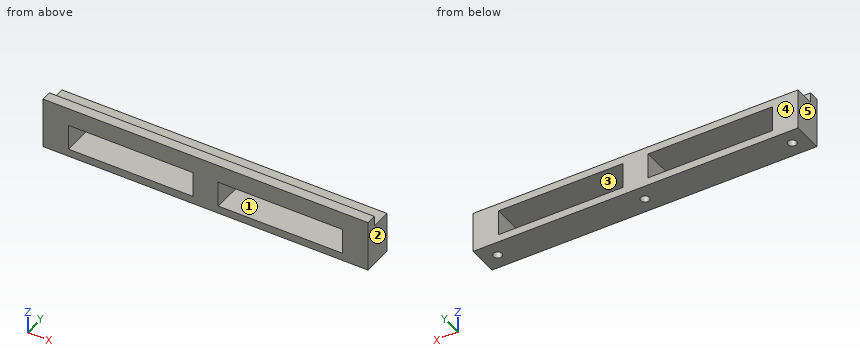
```python
from build123d import *

# Parameters (mm, degrees)
F0_W     = 101.6
F0_H     = 9.525
F1_DEPTH = 12.762509
F2_W     = 101.6
F2_H     = 3.175
F3_DEPTH = 3.175
F4_W     = 38.89375
F4_H     = 8.000009
F5_DEPTH = 9.525
F6_R     = 1.35255
F7_DEPTH = 10.381259


with BuildPart() as f1:
    # F0 (on Top) → F1 (new body)
    with BuildSketch(Plane.XY):
        with Locations((50.8, -4.7625)):
            Rectangle(F0_W, F0_H)
    extrude(amount=F1_DEPTH)

    # F2 (on face) → F3 (join)
    with BuildSketch(Plane.XY.offset(12.762509)):
        with Locations((50.8, -7.9375)):
            Rectangle(F2_W, F2_H)
    extrude(amount=F3_DEPTH)

    # F4 (on face) → F5 (cut, through all)
    with BuildSketch(Plane(origin=(0, 0, 0), x_dir=(-1, 0, 0), z_dir=(0, 1, 0))):
        with Locations((-74.215625, 6.381254)):
            Rectangle(F4_W, F4_H)
        with Locations((-27.384375, 6.381254)):
            Rectangle(F4_W, F4_H)
    extrude(amount=-F5_DEPTH, mode=Mode.SUBTRACT)

    # F6 (on face) → F7 (cut, through all)
    with BuildSketch(Plane(origin=(0, 0, 0), x_dir=(1, 0, 0), z_dir=(0, 0, -1))):
        with Locations((96.8375, 4.7625)):
            Circle(F6_R)
        with Locations((50.8, 4.7625)):
            Circle(F6_R)
        with Locations((4.7625, 4.7625)):
            Circle(F6_R)
    extrude(amount=-F7_DEPTH, mode=Mode.SUBTRACT)


solid = f1.part
```
The listing builds one solid part. Answer for the finished solid, in the listing's coordinates (mm). Face numbers are marked on the shaded views. A direction names the side the tool comes from. Round coordinates to 2 decimals unless told otherwise and drop trailing zeros. Loops run counter-clockwise (first coordinate to the right, second up) from the corner with the lowest first, then second, coordinate; pieces in that order, holes last.
Q1. Find the intervals of material crossed by line 1 (X direction, y = -1, z = 4.5); line 2 (Z direction, x = 13.5, y = -8.5); line 3 (Z direction, x = 86, y = -1.75), in increasing order.
Q2. Section C-C, the plane z = 3.5 is taken. Determine the outline of the cut face in (x, y) (1 decimal).
Q3. Given pin 1 Ø1.5 at (x, y) = (75.5, -2) entering from -Z; pin 2 Ø1.4 at (x, y) = (96.5, -5) entering from -Z; pin 3 Ø3 at (x, y) = (86.5, -3) entering from +Z, each flat-ended and moving along its own axis, determine where each tip first touches the part or whether it passes through.
Q4. For a pull along X with two mould halves and no side action, classify the marked faces 3, 4 and 5 as released by +X, released by -X, zero draft, split by the parting line, or undercut.
Q5. Section B-B, the plane y = -2.5 is taken. Determine the outline of the cut face in (x, z).
Q6. Which of the six approach directions +Z, -Z, +X, -X, +Y, -Y give full straight-line access (tool end or side, diameter ignored) to the marked faces 1 and 2?
Completed:
1. line 1: x = 0 to 7.94, 46.83 to 54.77, 93.66 to 101.6
1. line 2: z = 0 to 2.38, 10.38 to 15.94
1. line 3: z = 0 to 2.38, 10.38 to 12.76
2. outline: (0, -9.5) - (7.9, -9.5) - (7.9, 0) - (0, 0) - close; (46.8, -9.5) - (54.8, -9.5) - (54.8, 0) - (46.8, 0) - close; (93.7, -9.5) - (101.6, -9.5) - (101.6, 0) - (93.7, 0) - close; hole circle Ø2.7 at (4.8, -4.8); hole circle Ø2.7 at (50.8, -4.8); hole circle Ø2.7 at (96.8, -4.8)
3. pin 1: stops at z = 0
3. pin 2: stops at z = 10.38
3. pin 3: stops at z = 12.76
4. face 3: undercut
4. face 4: zero draft
4. face 5: released by -X
5. outline: (0, 0) - (101.6, 0) - (101.6, 12.76) - (0, 12.76) - close; hole (7.94, 2.38) - (46.83, 2.38) - (46.83, 10.38) - (7.94, 10.38) - close; hole (54.77, 2.38) - (93.66, 2.38) - (93.66, 10.38) - (54.77, 10.38) - close
6. face 1: +Y, -Y
6. face 2: +Z, -Z, +X, +Y, -Y
